Verification items for the finished model (mm, model axes). Give positions to 0.01 mm unless a question says otherwise; leave off trailing zeros. Write each loop counter-clockwise with the first axis right and the second up, starting at its lowest first coordinate (ties: lowest second). Pieces come first, ordered by that corner, then holes. Notation, with made-up numbers: (59.25, 32) -> (116.25, 32) arc R21 ccw to (116.25, 66) -> close; hole circle Ø7 at (70.25, -35.75). An arc over 180 degrees is marked (long way). Answer as CSV lines item,"result". Start each with the question number.
1) Material ranges on L1, parallel to Y at x = 3.75, z = 0.2; L2, parallel to X at y = 5, z = 0.75; L3, parallel to X at y = 9.25, z = 8, recorded low to high.
2) Gauge pin test, flat ends, axial feed: pin 1 Ø2 at (x, y) = (-23.5, 6) entering from +Z; pin 2 Ø4 at (x, y) = (3.5, 7.5) entering from +Z; pin 3 Ø0.5 at (x, z) = (1, 0.5) entering from -Y; pin 4 Ø3 at (x, y) = (3.75, 6.27) entering from -Z. Record the tip position at first contact, or that the pin passes through.
3) Sectioned sample at B-B on y = 3.5. Record the cut outline in (x, z), and give its area (3 significant figures).
4) Sectioned sample at A-A on x = -20. Record the cut outline in (y, z), and give its area (3 significant figures).
5) Mould release check, pull along Y, two halves, no side actions. Record for faces 1 (the cylindrical face through (7.517, 6.361, 0.493)), 2 (the flat face through (0, 9, 6)), 3 (the cylindrical face through (4.488, 4.854, 0.493)): released by +Y, released by -Y, zero draft, split by the parting line, or undercut.
```python
from build123d import *

# Parameters (mm, degrees)
SKETCH1_R           = 1.6
BOSS_EXTRUDE1_DEPTH = 1
BOSS_EXTRUDE2_DEPTH = 15.492796704
SKETCH2_R           = 2
CUT_EXTRUDE2_DEPTH  = 43.166654476
CUT_EXTRUDE3_START  = -1.5
SKETCH2_3_R         = 2
CUT_EXTRUDE3_DEPTH  = 41.666654476
SKETCH3_W           = 29.5
SKETCH3_H           = 22.485495194
CUT_EXTRUDE4_DEPTH  = 43.166654476


with BuildPart() as part:
    # Sketch1 → Boss-Extrude1 (new body)
    # profile 1 of 3: a face of its own
    with BuildSketch(Plane.XY):
        Polygon((-29.5, 10.023123532), (-29.5, 13), (0, 13), (0, 10.023123532), (0, 2.523123532), (0, 0), (-29.5, 0), (-29.5, 2.523123532), align=None)
    # profile 2 of 3: a face of its own
    with BuildSketch(Plane.XY):
        with BuildLine():
            ThreePointArc((3.38, 10.023123532), (7.518209124, 6.273123532), (3.38, 2.523123532))
            Line((3.38, 2.523123532), (0, 2.523123532))
            Line((0, 2.523123532), (0, 10.023123532))
            Line((0, 10.023123532), (3.38, 10.023123532))
        make_face()
        with Locations((3.75, 6.273123532)):
            Circle(SKETCH1_R, mode=Mode.SUBTRACT)
    # profile 3 of 3: a face of its own
    with BuildSketch(Plane.XY):
        with BuildLine():
            ThreePointArc((-32.88, 2.541421507), (-37, 6.273123532), (-32.88, 10.004825556))
            Line((-32.88, 10.004825556), (-29.5, 10.023123532))
            Line((-29.5, 10.023123532), (-29.5, 2.523123532))
            Line((-29.5, 2.523123532), (-32.88, 2.541421507))
        make_face()
        with Locations((-33.25, 6.273123532)):
            Circle(SKETCH1_R, mode=Mode.SUBTRACT)
    extrude(amount=BOSS_EXTRUDE1_DEPTH)

    # Sketch1<4> → Boss-Extrude2 (add)
    with BuildSketch(Plane.XY):
        Polygon((-29.5, 10.023123532), (-29.5, 13), (0, 13), (0, 10.023123532), (0, 2.523123532), (0, 0), (-29.5, 0), (-29.5, 2.523123532), align=None)
    extrude(amount=BOSS_EXTRUDE2_DEPTH)

    # Sketch2 → Cut-Extrude2 (cut, through all)
    with BuildSketch(Plane(origin=(0, 0, 0), x_dir=(1, 0, 0), z_dir=(0, -0.7660444431189791, 0.642787609686538))):
        with Locations(Location((-4.75, 15.224409749, 0), (0, 0, 270))):
            Circle(SKETCH2_R)
        with Locations(Location((-24.75, 15.224409749, 0), (0, 0, 270))):
            Circle(SKETCH2_R)
    extrude(amount=-CUT_EXTRUDE2_DEPTH, mode=Mode.SUBTRACT)

    # Sketch2<3> → Cut-Extrude3 (cut, through all)
    # profile 1 of 2: a face of its own
    with BuildSketch(Plane(origin=(0, 0, 0), x_dir=(1, 0, 0), z_dir=(0, -0.7660444431189791, 0.642787609686538)).offset(CUT_EXTRUDE3_START)):
        Polygon((-2.787009085, 11.824409749), (-0.82401817, 15.224409749), (-2.787009085, 18.624409749), (-6.712990915, 18.624409749), (-8.67598183, 15.224409749), (-6.712990915, 11.824409749), align=None)
        with Locations(Location((-4.75, 15.224409749, 0), (0, 0, 270))):
            Circle(SKETCH2_3_R, mode=Mode.SUBTRACT)
    # profile 2 of 2: a face of its own
    with BuildSketch(Plane(origin=(0, 0, 0), x_dir=(1, 0, 0), z_dir=(0, -0.7660444431189791, 0.642787609686538)).offset(CUT_EXTRUDE3_START)):
        Polygon((-20.82401817, 15.224409749), (-22.787009085, 18.624409749), (-26.712990915, 18.624409749), (-28.67598183, 15.224409749), (-26.712990915, 11.824409749), (-22.787009085, 11.824409749), align=None)
        with Locations(Location((-24.75, 15.224409749, 0), (0, 0, 270))):
            Circle(SKETCH2_3_R, mode=Mode.SUBTRACT)
    extrude(amount=-CUT_EXTRUDE3_DEPTH, mode=Mode.SUBTRACT)

    # Sketch3 → Cut-Extrude4 (cut, through all)
    with BuildSketch(Plane(origin=(0, 0, 0), x_dir=(1, 0, 0), z_dir=(0, -0.7660444431189791, 0.642787609686538))):
        with Locations((-14.75, 8.981662152)):
            Rectangle(SKETCH3_W, SKETCH3_H)
    extrude(amount=CUT_EXTRUDE4_DEPTH, mode=Mode.SUBTRACT)


solid = part.part
```
Ans:
1,L1,"y = 2.5 to 4.67, 7.87 to 10.04"
1,L2,"x = -36.78 to -34.22, -32.28 to 2.78, 4.72 to 7.3"
1,L3,"x = -29.5 to -26.86, -22.64 to -6.86, -2.64 to 0"
2,pin 1,"stops at z = 8.34"
2,pin 2,"stops at z = 1"
2,pin 3,"stops at y = 2.52"
2,pin 4,"passes through"
3,outline,"(-35.77, 0) -> (6.3, 0) -> (6.3, 1) -> (0, 1) -> (0, 4.17) -> (-29.5, 4.17) -> (-29.5, 1) -> (-35.77, 1) -> close"
3,area,"136 mm²"
4,outline,"(0, 0) -> (13, 0) -> (13, 15.49) -> close"
4,area,"101 mm²"
5,face 1,"split by the parting line"
5,face 2,"zero draft"
5,face 3,"undercut"
